Can you work these out from the model? Positions are in its coordinate system, mm. A direction names the side the tool comes from. Coordinates: 2 decimals unless noted, no trailing zeros. Loops run counter-clockwise (first coordinate to the right, second up) from the corner with the lowest first, then second, coordinate; pieces in that order, holes last.
```python
from build123d import *

# Parameters (mm, degrees)
F0_R           = 12.7
F1_DEPTH       = 6.35
F3_DEPTH       = 3.175
F4_R           = 5.55625
F5_DEPTH       = 3.175
F6_R           = 3.96875
F7_DEPTH       = 8.73125
F8_R           = 2.2479
F9_DEPTH       = 15.08125
F11_DEPTH      = 6.35
F12_COUNT      = 12
F12_ANGLE      = 330
F14_END_RADIUS = 5.55625
F14_REACH      = 18.1506366107
F17_END_RADIUS = 5.55625
F17_REACH      = 35.6755158286


with BuildPart() as f1:
    # F0 (on Top) → F1 (new body)
    with BuildSketch(Plane.XY):
        Circle(F0_R)
    extrude(amount=F1_DEPTH)

    # F2 (on face) → F3 (cut)
    with BuildSketch(Plane(origin=(0, 0, 0), x_dir=(1, 0, 0), z_dir=(0, 0, -1))):
        Polygon((2.6100007461, 4.5206539), (-2.6100007461, 4.5206539), (-5.2200014922, 0), (-2.6100007461, -4.5206539), (2.6100007461, -4.5206539), (5.2200014922, 0), align=None)
    extrude(amount=-F3_DEPTH, mode=Mode.SUBTRACT)

    # F4 (on face) → F5 (join)
    with BuildSketch(Plane.XY.offset(6.35)):
        Circle(F4_R)
    extrude(amount=F5_DEPTH)

    # F6 (on face) → F7 (join)
    with BuildSketch(Plane.XY.offset(9.525)):
        Circle(F6_R)
    extrude(amount=F7_DEPTH)

    # F8 (on face) → F9 (cut, through all)
    with BuildSketch(Plane(origin=(0, 0, 3.175), x_dir=(1, 0, 0), z_dir=(0, 0, -1))):
        Circle(F8_R)
    extrude(amount=-F9_DEPTH, mode=Mode.SUBTRACT)

    # F10 (on face) → F11 (join, through all)
    with BuildSketch(Plane(origin=(0, 0, 0), x_dir=(1, 0, 0), z_dir=(0, 0, -1))):
        with BuildLine():
            ThreePointArc((-1.5843963802, 12.60078125), (0, 12.7), (1.5843963802, 12.60078125))
            ThreePointArc((1.5843963802, 12.60078125), (0, 14.2875), (-1.5843963802, 12.60078125))
        make_face()
    f11 = extrude(amount=-F11_DEPTH)

    # F12: F11 ×12 about axis
    f12_axis = Axis((0, 0, 0), (0, 0, -1))
    for i in range(1, F12_COUNT):
        add(f11.rotate(f12_axis, i * F12_ANGLE / (F12_COUNT - 1)))

    f14_end = (Plane(origin=(0, 0, 7.9375), x_dir=(-1, 0, 0), z_dir=(0, 0, -1)) * Cylinder(F14_END_RADIUS, 124.9884067655, mode=Mode.PRIVATE)).faces().sort_by_distance((-5.55625, 0, 7.9375))[0]
    # F13 (on Front) → F14 (cut, up to the whole of a round face its end follows)
    with BuildSketch(Plane.XZ):
        with BuildLine():
            ThreePointArc((0, 8.0772), (-1.7272, 6.35), (0, 4.6228))
            Line((0, 4.6228), (0, 8.0772))
        make_face()
        with BuildLine():
            Line((0, 8.0772), (0, 4.6228))
            ThreePointArc((0, 4.6228), (1.2213148325, 5.1286851675), (1.7272, 6.35))
            ThreePointArc((1.7272, 6.35), (1.2213148325, 7.5713148325), (0, 8.0772))
        make_face()
    f14_long = extrude(amount=F14_REACH, mode=Mode.PRIVATE)
    add(split(f14_long, bisect_by=f14_end, keep=Keep.BOTTOM, mode=Mode.PRIVATE), mode=Mode.SUBTRACT)

    f17_end = (Plane(origin=(0, 0, 7.9375), x_dir=(-1, 0, 0), z_dir=(0, 0, -1)) * Cylinder(F17_END_RADIUS, 160.0381652835, mode=Mode.PRIVATE)).faces().sort_by_distance((-5.55625, 0, 7.9375))[0]
    # F16 (on offset) → F17 (cut, up to the whole of a round face its end follows)
    with BuildSketch(Plane.XZ.offset(14.2875)):
        with BuildLine():
            Line((3.175, 6.35), (-3.175, 6.35))
            ThreePointArc((-3.175, 6.35), (0, 3.175), (3.175, 6.35))
        make_face()
    f17_long = extrude(amount=-F17_REACH, mode=Mode.PRIVATE)
    add(split(f17_long, bisect_by=f17_end, keep=Keep.ALL, mode=Mode.PRIVATE).solids().sort_by_distance((0, -14.2875, 5.0024881485))[0], mode=Mode.SUBTRACT)


solid = f1.part
```
Item 1: Suppose I cut it at A-A, the plane y = -2.75. Please give me the cut outline in (x, z) (3 decimals).
Results are:
outline: (-12.399, 0) - (-3.632, 0) - (-3.632, 3.175) - (3.632, 3.175) - (3.632, 0) - (12.399, 0) - (12.399, 6.35) - (4.828, 6.35) - (4.828, 9.525) - (2.862, 9.525) - (2.862, 18.256) - (-2.862, 18.256) - (-2.862, 9.525) - (-4.828, 9.525) - (-4.828, 6.35) - (-12.399, 6.35) - close; hole circle Ø3.454 at (0, 6.35)
Item 2: I need wall thicknesses on line 1 along X through (y, z) = (0, 7); line 2 along Y through (x, z) = (0, 10.5); line 3 along X through (y, z) = (0, 2.75). Which ranges of each line are inside material? Lowest first, please.
Results are:
line 1: x = -5.56 to -2.25, 2.25 to 5.56
line 2: y = -3.97 to -2.25, 2.25 to 3.97
line 3: x = -14.29 to -5.22, 5.22 to 14.29
Item 3: I'm going to push flat-ended pins straight in: P1, Ø5, axis at y = 3, z = 10, coming from the -X side; P2, Ø8, axis at x = -1.5, z = 11.5, coming from the +Y side; P3, Ø1, axis at x = -3.5, y = -5, coming from the +Z side. Where does each tip first touch, or does it pass through?
Results are:
P1: stops at x = -5.53
P2: stops at y = 5.56
P3: stops at z = 6.35
Item 4: Suppose I cut it at C-C, the plane x = -0.75. Please give me the cut outline in (y, z) (3 decimals), plus the area to 3 significant figures.
Results are:
outline: (-14.099, 0) - (-4.521, 0) - (-4.521, 3.175) - (-2.119, 3.175) - (-2.119, 4.794) - (-5.505, 4.794) - (-5.505, 3.265) - (-14.099, 3.265) - close; (-5.505, 7.906) - (-2.119, 7.906) - (-2.119, 18.256) - (-3.897, 18.256) - (-3.897, 9.525) - (-5.505, 9.525) - close; (2.119, 3.175) - (4.521, 3.175) - (4.521, 0) - (14.099, 0) - (14.099, 6.35) - (5.505, 6.35) - (5.505, 9.525) - (3.897, 9.525) - (3.897, 18.256) - (2.119, 18.256) - close
area: 152 mm2
Item 5: Suppose I cut it at B-B, the plane z = 11.25. Please give me the cut outline in (x, y), plus the area to 3 significant figures.
Results are:
outline: circle Ø7.94 at (0, 0); hole circle Ø4.5 at (0, 0)
area: 33.6 mm2
Item 6: Suppose I cut it at D-D, the plane y = 6.35. Please give me the cut outline in (x, z).
Results are:
outline: (-12.59, 0) - (12.59, 0) - (12.59, 6.35) - (-12.59, 6.35) - close
Item 7: On a 3-axis mill with a long thin cutter (end or side, diameter ignored), from which of +Z, -Z, +X, -X, +Y, -Y can I reach the whole of each face in a straight line? I mean faces 1 (the face through (3.264, -12.274, 2.425)), 2 (the face through (2.56, -4.93, 7.72)), 3 (the face through (0, 4.521, 2)), 4 (the face through (-0.07, -9.492, 3.176)). Say none if no direction works.
Results are:
face 1: +Z, -Z, -Y
face 2: +Z
face 3: -Z
face 4: +Z, -Y
Item 8: We'd pull the mould along X, two halves only. Please class faces 5 (the face through (12.391, -7.112, 3.131)), 6 (the face through (-7.112, -12.391, 3.131)), 7 (the face through (-0.86, -3.874, 13.83)), 8 (the face through (-4, 1, 9.525)): +X half, -X half, draft (parallel to the pull), parting line (faces both ways), or undercut.
Results are:
face 5: undercut
face 6: undercut
face 7: parting line
face 8: draft
